Autodesk Inventor part; units mm, degrees
ref_plane "YZ Plane" through (0, 0, 0) normal (1, 0, 0) x (0, 1, 0)
ref_plane "XZ Plane" through (0, 0, 0) normal (0, 1, 0) x (-1, 0, 0)
ref_plane "XY Plane" through (0, 0, 0) normal (0, 0, 1) x (1, 0, 0)
sketch "Sketch2" plane through (0, 0, 0) normal (0, 1, 0) x (-1, 0, 0)
  line L0 (-39, 86) -> (39, 86)
  arc A0 (43, 82) -> (39, 86) centre (39, 82) ccw
  line L1 (43, 82) -> (43, -66)
  arc A1 (39, -70) -> (43, -66) centre (39, -66) ccw
  line L2 (39, -70) -> (-39, -70)
  arc A2 (-43, -66) -> (-39, -70) centre (-39, -66) ccw
  line L3 (-43, -66) -> (-43, 82)
  arc A3 (-39, 86) -> (-43, 82) centre (-39, 82) ccw
  circle A4 centre (-36.5, 79.5) radius 1.5
  circle A5 centre (36.5, 79.5) radius 1.5
  circle A6 centre (-36.5, -63.5) radius 1.5
  circle A7 centre (36.5, -63.5) radius 1.5
  line L4 (-30, 61) -> (-27.5, 61)
  line L5 (-30, 61) -> (-25, 41)
  line L6 (-25, 61) -> (-20, 41)
  line L7 (-20, 61) -> (-15, 41)
  line L8 (-15, 61) -> (-10, 41)
  line L9 (-10, 61) -> (-5, 41)
  line L10 (-5, 61) -> (-1.5, 47)
  line L11 (30, 61) -> (25, 41)
  line L12 (25, 61) -> (20, 41)
  line L13 (20, 61) -> (15, 41)
  line L14 (15, 61) -> (10, 41)
  line L15 (10, 61) -> (5, 41)
  line L16 (5, 61) -> (1.5, 47)
  line L17 (-20, 61) -> (-17.5, 61)
  line L18 (-22.5, 41) -> (-25, 41)
  line L19 (-10, 61) -> (-7.5, 61)
  line L20 (-12.5, 41) -> (-15, 41)
  line L21 (25, 41) -> (22.5, 41)
  line L22 (27.5, 61) -> (30, 61)
  line L23 (15, 41) -> (12.5, 41)
  line L24 (17.5, 61) -> (20, 61)
  line L25 (7.5, 61) -> (10, 61)
  line L26 (22.5, 41) -> (27.5, 61)
  line L27 (20, 41) -> (17.5, 41)
  line L28 (25, 61) -> (22.5, 61)
  line L29 (17.5, 41) -> (22.5, 61)
  line L30 (12.5, 41) -> (17.5, 61)
  line L31 (15, 61) -> (12.5, 61)
  line L32 (10, 41) -> (7.5, 41)
  line L33 (7.5, 41) -> (12.5, 61)
  line L34 (-22.5, 41) -> (-27.5, 61)
  line L35 (-12.5, 41) -> (-17.5, 61)
  line L36 (-22.5, 61) -> (-25, 61)
  line L37 (-17.5, 41) -> (-20, 41)
  line L38 (-17.5, 41) -> (-22.5, 61)
  line L39 (-7.5, 41) -> (-10, 41)
  line L40 (-12.5, 61) -> (-15, 61)
  line L41 (-7.5, 41) -> (-12.5, 61)
  line L42 (2.5, 41) -> (7.5, 61)
  line L43 (-2.5, 41) -> (-7.5, 61)
  line L44 (5, 41) -> (2.5, 41)
  line L45 (-2.5, 41) -> (-5, 41)
  line L46 (5, 61) -> (1.5, 61)
  line L47 (1.5, 61) -> (1.5, 47)
  line L48 (-5, 61) -> (-1.5, 61)
  line L49 (-1.5, 61) -> (-1.5, 47)
  circle A8 centre (15, 18) radius 2.5
  circle A9 centre (0, 18) radius 2.5
  circle A10 centre (-15, 18) radius 2.5
  circle A11 centre (10, -40) radius 8
  circle A12 centre (-10, -40) radius 8
  circle A13 centre (20, -20) radius 8
  circle A14 centre (0, -20) radius 8
  circle A15 centre (-20, -20) radius 8
  circle A16 centre (20, 0) radius 8
  circle A17 centre (0, 0) radius 8
  circle A18 centre (-20, 0) radius 8
  point P0 (-43, -66)
  point P1 (39, -70)
  point P2 (43, 82)
  dimension "d6" = 3.5
  dimension "d7" = 3.5
  dimension "d8" = 90
  dimension "d10" = 5
  dimension "d11" = 5
  dimension "d12" = 5
  dimension "d13" = 16
  dimension "d14" = 16
  dimension "d15" = 16
  dimension "d16" = 16
  dimension "d17" = 16
  dimension "d18" = 16
  dimension "d19" = 16
  dimension "d20" = 16
extrude "Extrusion2" add sketch "Sketch2" along normal blind 3
fillet "Fillet2" radius 1.5 8 edges at (41.8284, 3, -68.8284) (0, 3, -70) (-41.8284, 3, -68.8284) (-43, 3, 8) (-41.8284, 3, 84.8284) (0, 3, 86) (41.8284, 3, 84.8284) (43, 3, 8)
properties part number "TUTUP CASING"
Check sheet for the modelled part. Datum: model origin and axes. Units: mm. A direction names the side the tool comes from. Round coordinates to 2 decimals unless told otherwise and drop trailing zeros. Order: outer loops, then holes, each group sorted by start corner. A loop starts at its lowest first (then second) coordinate and runs counter-clockwise, first axis right, second up. Notation, with made-up numbers: (-0.5, 58.5) -> (22.5, 58.5) arc R33 cw to (22.5, 95.5) -> close; hole circle Ø5 at (-8.5, 86). An arc over 180 degrees is marked (long way). One line per item, written item: value. Start each with the question number.
Q1. Gauge pin test, flat end, axial feed: pin 1 Ø9.5 at (x, z) = (-20, -20) entering from +Y. Record the tip position at first contact, or that the pin passes through.
Q2. Cross-section at C-C (x = 36.5). Record the boundary of the cut face in (y, z), and give its area (3 significant figures).
Q3. Cross-section at D-D (z = -63.5). Record the boundary of the cut face in (x, y).
Q4. Cross-section at B-B (z = 0). Record the boundary of the cut face in (x, y).
Q5. Set-up check for faces 1 (the face through (-3, 1, 61)), 2 (the face through (41.797, 0.74, -68.859)): record each of +Z, -Z, +X, -X, +Y, -Y from which the full face is reachable in a straight line by a thin tool's end or side.
Q6. Cross-section at A-A (x = 0). Record the boundary of the cut face in (y, z).
Q7. Thickness scan on line 1 (Z direction, x = 36.5, y = 1.85); line 2 (X direction, y = 1.05, z = -45) (3 decimals); line 3 (X direction, y = 2.2, z = 79.5). Record the ranges inside material, lowest first.
Completed:
1. pin 1: passes through
2. outline: (0, -70) -> (1.5, -70) arc R1.5 ccw to (3, -68.5) -> (3, -65) -> (0, -65) -> close; (0, -62) -> (3, -62) -> (3, 78) -> (0, 78) -> close; (0, 81) -> (3, 81) -> (3, 84.5) arc R1.5 ccw to (1.5, 86) -> (0, 86) -> close
2. area: 449 mm²
3. outline: (-43, 0) -> (-38, 0) -> (-38, 3) -> (-41.5, 3) arc R1.5 ccw to (-43, 1.5) -> close; (-35, 0) -> (35, 0) -> (35, 3) -> (-35, 3) -> close; (38, 0) -> (43, 0) -> (43, 1.5) arc R1.5 ccw to (41.5, 3) -> (38, 3) -> close
4. outline: (-43, 0) -> (-28, 0) -> (-28, 3) -> (-41.5, 3) arc R1.5 ccw to (-43, 1.5) -> close; (-12, 0) -> (-8, 0) -> (-8, 3) -> (-12, 3) -> close; (8, 0) -> (12, 0) -> (12, 3) -> (8, 3) -> close; (28, 0) -> (43, 0) -> (43, 1.5) arc R1.5 ccw to (41.5, 3) -> (28, 3) -> close
5. face 1: +Y, -Y
5. face 2: -Z, +X, +Y, -Y
6. outline: (0, -70) -> (1.5, -70) arc R1.5 ccw to (3, -68.5) -> (3, -28) -> (0, -28) -> close; (0, -12) -> (3, -12) -> (3, -8) -> (0, -8) -> close; (0, 8) -> (3, 8) -> (3, 15.5) -> (0, 15.5) -> close; (0, 20.5) -> (3, 20.5) -> (3, 84.5) arc R1.5 ccw to (1.5, 86) -> (0, 86) -> close
7. line 1: z = -69.96 to -65, -62 to 78, 81 to 85.96
7. line 2: x = -43 to -16.245, -3.755 to 3.755, 16.245 to 43
7. line 3: x = -42.83 to -38, -35 to 35, 38 to 42.83
